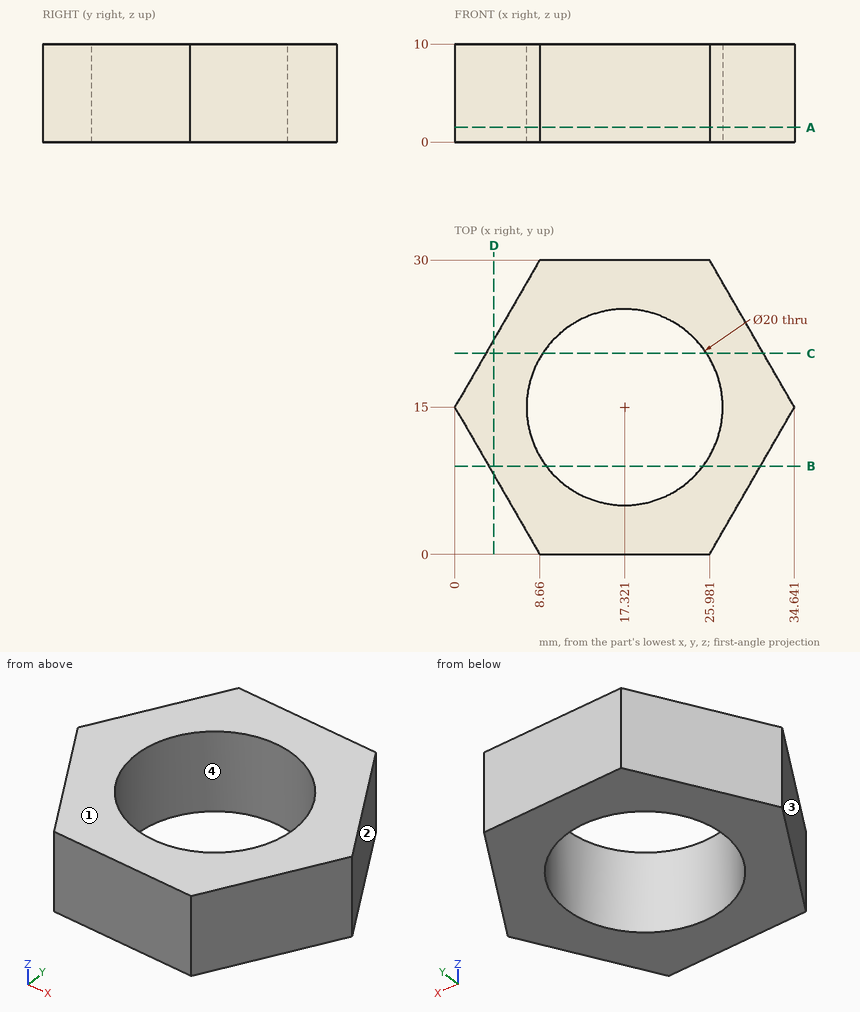
Geometry: see drawing. Coordinates: mm, zero at the bounding-box minimum. Give positions to 0.01 mm unless a question says otherwise; leave off trailing zeros. Loops run counter-clockwise (first coordinate to the right, second up) from the corner with the lowest first, then second, coordinate; pieces in that order, holes last. Notation, with made-up numbers: (75.5, -2.5) - (80.5, -2.5) arc R21 ccw to (80.5, 32.5) - close; hole circle Ø6 at (-0.75, 85.25). An arc over 180 degrees is marked (long way). Use CSV: the item, a comma, the result in double quotes. Start each with the question number.
Item 1: Section B-B on y = 9. Return loops of the section in (x, z) (1 decimal).
Item 2: Mould query, pull axis X, two halves, no side actions, for the marked faces 1, 2, 3 and 4. Classes: pulls with the +X half, pulls with the -X half, needs draft (parallel to the pull), parting line crosses it, or undercut.
Item 3: Line query: line 1 (Y direction, x = 15, z = 1.25); line 2 (X direction, y = 12.5, z = 5.5) (1 decimal); line 3 (X direction, y = 19, z = 5) (1 decimal). Output: solid intervals per line, ascending.
Item 4: Section A-A on z = 1.5. Return loops of the section in (x, y).
Item 5: Contact query for flat-ended pins moving along their axis: P1, Ø1, axis at x = 9.5, y = 25.5, coming from the -Z side; P2, Ø16, axis at x = 17.32, y = 15, coming from the -Z side; P3, Ø1.5, axis at y = 26, z = 5, coming from the +X side; P4, Ø6, axis at y = 16.5, z = 4, coming from the +X side. Output: stop coordinate, or through.
Item 6: Section D-D on x = 4. Return loops of the section in (y, z), then the cut area to 3 significant figures.
Item 7: Section C-C on y = 20.5. Return loops of the section in (x, z) (1 decimal).
Ans:
1,outline,"(3.5, 0) - (9.3, 0) - (9.3, 10) - (3.5, 10) - close; (25.3, 0) - (31.2, 0) - (31.2, 10) - (25.3, 10) - close"
2,face 1,"needs draft"
2,face 2,"pulls with the +X half"
2,face 3,"pulls with the -X half"
2,face 4,"undercut"
3,line 1,"y = 0 to 5.27, 24.73 to 30"
3,line 2,"x = 1.4 to 7.6, 27 to 33.2"
3,line 3,"x = 2.3 to 8.2, 26.5 to 32.3"
4,outline,"(0, 15) - (8.66, 0) - (25.98, 0) - (34.64, 15) - (25.98, 30) - (8.66, 30) - close; hole circle Ø20 at (17.32, 15)"
5,P1,"stops at z = 0"
5,P2,"passes through"
5,P3,"stops at x = 28.72"
5,P4,"stops at x = 34.64"
6,outline,"(8.07, 0) - (21.93, 0) - (21.93, 10) - (8.07, 10) - close"
6,area,"139 mm2"
7,outline,"(3.2, 0) - (9, 0) - (9, 10) - (3.2, 10) - close; (25.7, 0) - (31.5, 0) - (31.5, 10) - (25.7, 10) - close"
